Input: part model. Units: mm. Frame: model coordinates. A direction names the side the tool comes from. Coordinates: 2 decimals unless noted, no trailing zeros. Loops run counter-clockwise (first coordinate to the right, second up) from the corner with the lowest first, then second, coordinate; pieces in that order, holes last.
Item 1: Section B-B on x = -19. Return loops of the section in (y, z), and give its area (3 significant figures).
Item 2: Section C-C on z = 1.85. Return loops of the section in (x, y).
Item 3: Section D-D on y = -20. Return loops of the section in (x, z).
Item 4: Reachability of faces 1 (the cylindrical face through (-1.73, -7.81, 1.97)), 2 (the flat face through (-29.906, -39.288, 1.972)) from +Z, -Z, +X, -X, +Y, -Y: full face, straight path, thin tool, end or side. Return the list, or none.
Item 5: Section A-A on x = 0. Return loops of the section in (y, z).
Item 6: Contact query for a flat-ended pin moving along its axis: P1, Ø14.5, axis at x = 0, y = 0, coming from the +Z side. Output: stop coordinate, or through.
Item 7: Pull-direction query (X, two-part tool) for faces 3 (the cylindrical face through (-32, -49.01, 1.97)), 4 (the flat face through (10, 5, 4)), 5 (the cylindrical face through (38.489, 20.264, 1.972)); classes: released by +X, released by -X, zero draft, split by the parting line, or undercut.
Item 8: Ray query, line 1 along Y through (x, z) = (0, 2.95); line 2 along Y through (x, z) = (3.5, 2.3); line 3 along Y through (x, z) = (-7, 3.4). Return the intervals inside material, ascending.
```python
from build123d import *

# Parameters (mm, degrees)
SKETCH1_R           = 5.5
SKETCH1_R_2         = 8
BOSS_EXTRUDE1_DEPTH = 4


with BuildPart() as part:
    # Sketch1 → Boss-Extrude1 (new body)
    with BuildSketch(Plane.XY):
        with BuildLine():
            Line((-31.281072244, -42.237359284), (-28.491744654, -36.255626964))
            ThreePointArc((-28.491744654, -36.255626964), (-28.106649146, -33.233302048), (-29.547148474, -30.548584534))
            ThreePointArc((-29.547148474, -30.548584534), (-41.492580303, 9.198683592), (-13.868421053, 40.173584574))
            ThreePointArc((-13.868421053, 40.173584574), (-11.428274645, 41.997983641), (-10.5, 44.899888641))
            Line((-10.5, 44.899888641), (-10.5, 53.5))
            ThreePointArc((-10.5, 53.5), (0, 64), (10.5, 53.5))
            Line((10.5, 53.5), (10.5, 44.899888641))
            ThreePointArc((10.5, 44.899888641), (11.428274645, 41.997983641), (13.868421053, 40.173584574))
            ThreePointArc((13.868421053, 40.173584574), (26.601747568, 33.145090531), (36.219634513, 22.234839234))
            ThreePointArc((36.219634513, 22.234839234), (38.528932384, 20.247406269), (41.562966054, 19.969222638))
            Line((41.562966054, 19.969222638), (48.00662842, 21.397748193))
            ThreePointArc((48.00662842, 21.397748193), (60.530352441, 13.419256064), (52.551860313, 0.895532043))
            Line((52.551860313, 0.895532043), (46.108197947, -0.532993511))
            ThreePointArc((46.108197947, -0.532993511), (43.475995088, -2.067351539), (42.22298591, -4.844528963))
            ThreePointArc((42.22298591, -4.844528963), (26.601747568, -33.145090531), (-4.409032487, -42.270680531))
            ThreePointArc((-4.409032487, -42.270680531), (-7.39158054, -42.892897179), (-9.459281126, -45.130610461))
            Line((-9.459281126, -45.130610461), (-12.248608716, -51.112342781))
            ThreePointArc((-12.248608716, -51.112342781), (-13.414168685, -53.040091057), (-14.964105225, -54.674851032))
            Line((-14.964105225, -54.674851032), (-28.565575734, -54.674851032))
            ThreePointArc((-28.565575734, -54.674851032), (-32.023186029, -48.914571235), (-31.281072244, -42.237359284))
        make_face()
        with Locations((50.279244367, 11.146640118)):
            Circle(SKETCH1_R, mode=Mode.SUBTRACT)
        with Locations((0, 53.5)):
            Circle(SKETCH1_R, mode=Mode.SUBTRACT)
        with Locations((-21.76484048, -46.674851032)):
            Circle(SKETCH1_R, mode=Mode.SUBTRACT)
        Circle(SKETCH1_R_2, mode=Mode.SUBTRACT)
    extrude(amount=BOSS_EXTRUDE1_DEPTH)


solid = part.part
```
Results found:
1. outline: (-54.67, 0) - (-51.43, 0) - (-51.43, 4) - (-54.67, 4) - close; (-41.92, 0) - (38.02, 0) - (38.02, 4) - (-41.92, 4) - close
1. area: 333 mm2
2. outline: (-31.28, -42.24) arc R10.5 ccw to (-28.57, -54.67) - (-14.96, -54.67) arc R10.5 ccw to (-12.25, -51.11) - (-9.46, -45.13) arc R5 cw to (-4.41, -42.27) arc R42.5 ccw to (42.22, -4.84) arc R5 cw to (46.11, -0.53) - (52.55, 0.9) arc R10.5 ccw to (48.01, 21.4) - (41.56, 19.97) arc R5 cw to (36.22, 22.23) arc R42.5 ccw to (13.87, 40.17) arc R5 cw to (10.5, 44.9) - (10.5, 53.5) arc R10.5 ccw to (-10.5, 53.5) - (-10.5, 44.9) arc R5 cw to (-13.87, 40.17) arc R42.5 ccw to (-29.55, -30.55) arc R5 cw to (-28.49, -36.26) - close; hole circle Ø11 at (-21.76, -46.67); hole circle Ø16 at (0, 0); hole circle Ø11 at (0, 53.5); hole circle Ø11 at (50.28, 11.15)
3. outline: (-37.5, 0) - (37.5, 0) - (37.5, 4) - (-37.5, 4) - close
4. face 1: +Z, -Z
4. face 2: +Z, -Z, -X
5. outline: (-42.5, 0) - (-8, 0) - (-8, 4) - (-42.5, 4) - close; (8, 0) - (48, 0) - (48, 4) - (8, 4) - close; (59, 0) - (64, 0) - (64, 4) - (59, 4) - close
6. P1: passes through
7. face 3: released by -X
7. face 4: zero draft
7. face 5: undercut
8. line 1: y = -42.5 to -8, 8 to 48, 59 to 64
8. line 2: y = -42.36 to -7.19, 7.19 to 49.26, 57.74 to 63.4
8. line 3: y = -42.69 to -3.87, 3.87 to 61.33
